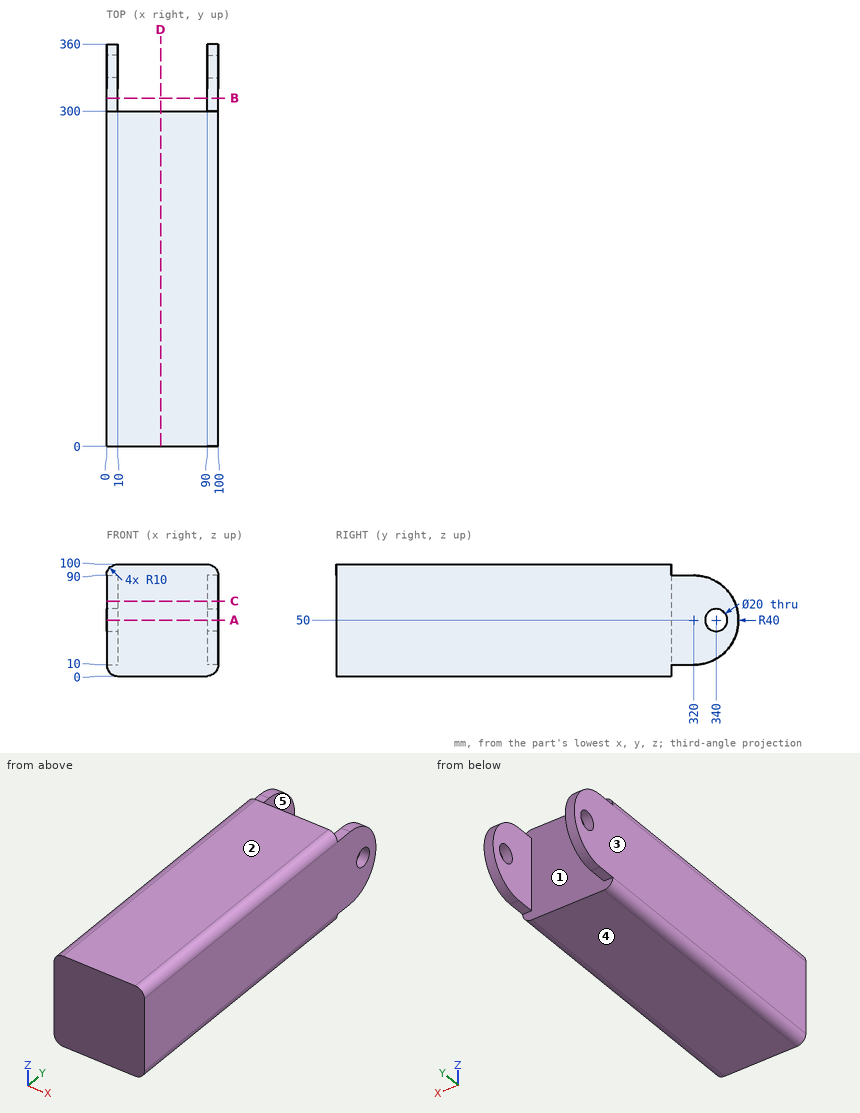
Job drawing, mm, ordinate dimensions from the low corner. One solid piece. A direction names the side the tool comes from. Coordinates: 2 decimals unless noted, no trailing zeros. Loops run counter-clockwise (first coordinate to the right, second up) from the corner with the lowest first, then second, coordinate; pieces in that order, holes last. Notation, with made-up numbers: (89.5, 9) -> (105.5, 9) arc R9 cw to (105.5, 21) -> close; hole circle Ø10 at (-2.75, -6.5). An arc over 180 degrees is marked (long way). One line per item, written item: value.
1. Slice it at C-C on z = 67. Write the cut outline in (x, y), and give its area (3 significant figures).
Answers:
outline: (0, 0) -> (100, 0) -> (100, 356.21) -> (90, 356.21) -> (90, 300) -> (10, 300) -> (10, 356.21) -> (0, 356.21) -> close
area: 31,100 mm^2
2. Slice it at D-D on x = 48.5. Write the cut outline in (y, z).
Answers:
outline: (0, 0) -> (300, 0) -> (300, 100) -> (0, 100) -> close
3. Slice it at A-A on z = 50. Write the cut outline in (x, y).
Answers:
outline: (0, 0) -> (100, 0) -> (100, 330) -> (90, 330) -> (90, 300) -> (10, 300) -> (10, 330) -> (0, 330) -> close; (0, 350) -> (10, 350) -> (10, 360) -> (0, 360) -> close; (90, 350) -> (100, 350) -> (100, 360) -> (90, 360) -> close
4. Pull direction X, two halves, no side cores. Call the marked faces 1, 2 and 3: pulls with the +X half, pulls with the -X half, needs draft (parallel to the pull), parting line crosses it, or undercut.
Answers:
face 1: undercut
face 2: needs draft
face 3: pulls with the -X half
5. Which spindle directions (+Z, -Z, +X, -X, +Y, -Y) get a long thin tool onto all of the face, cutting with end or side? Do the marked faces 4 and 5. Say none if no direction does.
Answers:
face 4: -Z, +X, -X, +Y, -Y
face 5: +Z, -Z, +Y
6. Drill centre lines: line 1 (Y direction, x = 93, z = 50); line 2 (X direction, y = 312, z = 75); line 3 (Y direction, x = 68.5, z = 19.5). Where is each one in solid material? Low to high. Write a range as [from, to].
Answers:
line 1: y = [0, 330], [350, 360]
line 2: x = [0, 10], [90, 100]
line 3: y = [0, 300]
7. Slice it at B-B on y = 311.5. Write the cut outline in (x, z).
Answers:
outline: (0, 10) -> (10, 10) -> (10, 90) -> (0, 90) -> close; (90, 10) -> (100, 10) -> (100, 90) -> (90, 90) -> close
8. Flat gauge pins, fed straight in: P1, Ø8, axis at x = 4.5, y = 314.5, coming from the +Z side; P2, Ø8, axis at x = 97, y = 305.5, coming from the -Z side; P3, Ø2, axis at x = 25.5, z = 81.5, coming from the +Y side. Where does each tip first touch, or does it go through?
Answers:
P1: stops at z = 90
P2: stops at z = 10
P3: stops at y = 300
